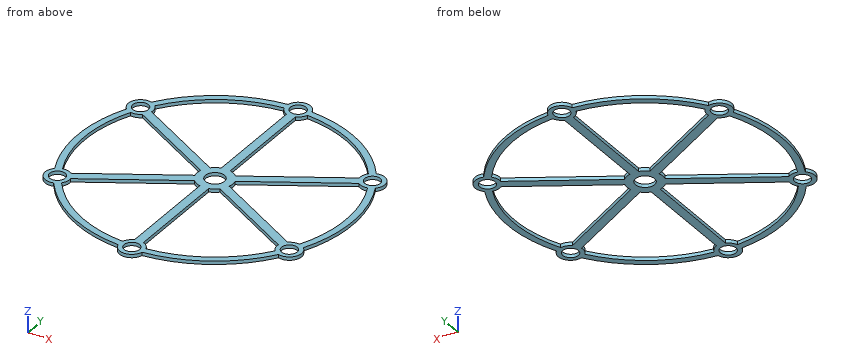
```python
from build123d import *

# Parameters (mm, degrees)
SKETCH_R           = 4.3
SKETCH_R_2         = 3.5
PAD_DEPTH          = 1.5
POLARPATTERN_COUNT = 6


with BuildPart() as part:
    # Sketch → Pad (new body)
    with BuildSketch(Plane.XY):
        with BuildLine():
            ThreePointArc((6.6323005804, 4.4735432278), (4.6158793486, 6.534038402), (2, 7.7459666924))
            Line((2, 7.7459666924), (2, 54.876524617))
            ThreePointArc((2, 54.876524617), (3.9880427931, 56.2124526827), (5.2197393691, 58.2667022995))
            ThreePointArc((48.4987282929, 32.7128052896), (29.7433833833, 50.3744520651), (5.2197393691, 58.2667022995))
            Line((48.4987282929, 32.7128052896), (50.9858410106, 34.390384))
            ThreePointArc((50.9858410106, 34.390384), (31.210195847, 52.9922463235), (5.3521454254, 61.2667041268))
            ThreePointArc((5.3521454254, 61.2667041268), (-3.6080213802, 64.1511663084), (-2, 54.876524617))
            Line((-2, 7.7459666924), (-2, 54.876524617))
            ThreePointArc((-2, 7.7459666924), (-2.8357963608, -7.4805253158), (6.6323005804, 4.4735432278))
        make_face()
        Circle(SKETCH_R, mode=Mode.SUBTRACT)
        with Locations((0, 60)):
            Circle(SKETCH_R_2, mode=Mode.SUBTRACT)
    pad = extrude(amount=PAD_DEPTH)

    # PolarPattern: Pad ×6 about axis
    polarpattern_axis = Axis((0, 0, 0), (0, 0, 1))
    for i in range(1, POLARPATTERN_COUNT):
        add(pad.rotate(polarpattern_axis, i * 360 / POLARPATTERN_COUNT))


solid = part.part
```
Part model, mm, in its own coordinate system. Round coordinates to 2 decimals unless told otherwise and drop trailing zeros. Write each loop counter-clockwise with the first axis right and the second up, starting at its lowest first coordinate (ties: lowest second). Pieces come first, ordered by that corner, then holes. Notation, with made-up numbers: (57.5, 45.5) -> (66.5, 45.5) arc R9 cw to (66.5, 54.5) -> close; hole circle Ø7 at (60.5, -17). An arc over 180 degrees is marked (long way). Return JSON: item names as keys, results as strings. Group by question number.
Q1. Saw through at B-B on x = 32.5. Write the cut outline in (y, z), plus the area to 3 significant figures.
Q2. Pin check, flat tips, straight feed: pin 1 (4 mm diameter, centred on x = -51.96, y = 30, fed in from +Z); pin 2 (0.8 mm diameter, centred on y = 34, z = 1, fed in from -X). Stop position of each tip, or through.
Q3. Saw through at D-D on y = 18.5. Write the cut outline in (x, z).
Q4. Saw through at C-C on y = -46. Write the cut outline in (x, z).
Q5. Probe L1, parallel to Y at x = 51.5, z = 0.7; L2, parallel to Y at x = -36.5, z = 1.35; L3, parallel to X at y = 9.5, z = 0.85. List the from-to ranges inside material, lowest first. Write a range as [from, to].
Q6. Saw through at A-A on y = 0. Write the cut outline in (x, z).
Answer:
{
 "1": {"outline": "(-52.21, 0) -> (-48.64, 0) -> (-48.64, 1.5) -> (-52.21, 1.5) -> close; (-21.07, 0) -> (-16.45, 0) -> (-16.45, 1.5) -> (-21.07, 1.5) -> close; (16.45, 0) -> (21.07, 0) -> (21.07, 1.5) -> (16.45, 1.5) -> close; (48.64, 0) -> (52.21, 0) -> (52.21, 1.5) -> (48.64, 1.5) -> close", "area": "24.6 mm2"},
 "2": {"pin 1": "through", "pin 2": "x = -56.12"},
 "3": {"outline": "(-58.65, 0) -> (-55.5, 0) -> (-55.5, 1.5) -> (-58.65, 1.5) -> close; (-36.04, 0) -> (-28.04, 0) -> (-28.04, 1.5) -> (-36.04, 1.5) -> close; (-2, 0) -> (2, 0) -> (2, 1.5) -> (-2, 1.5) -> close; (28.04, 0) -> (36.04, 0) -> (36.04, 1.5) -> (28.04, 1.5) -> close; (55.5, 0) -> (58.65, 0) -> (58.65, 1.5) -> (55.5, 1.5) -> close"},
 "4": {"outline": "(-40.82, 0) -> (-36.14, 0) -> (-36.14, 1.5) -> (-40.82, 1.5) -> close; (-2, 0) -> (2, 0) -> (2, 1.5) -> (-2, 1.5) -> close; (36.14, 0) -> (40.82, 0) -> (40.82, 1.5) -> (36.14, 1.5) -> close"},
 "5": {"L1": "[-35.48, -33.47], [-26.53, -24.52], [24.52, 26.53], [33.47, 35.48]", "L2": "[-49.5, -45.72], [-23.38, -18.76], [18.76, 23.38], [45.72, 49.5]", "L3": "[-60.76, -57.72], [-20.45, -12.45], [-2, 2], [12.45, 20.45], [57.72, 60.76]"},
 "6": {"outline": "(-61.5, 0) -> (-58.5, 0) -> (-58.5, 1.5) -> (-61.5, 1.5) -> close; (-8, 0) -> (-4.3, 0) -> (-4.3, 1.5) -> (-8, 1.5) -> close; (4.3, 0) -> (8, 0) -> (8, 1.5) -> (4.3, 1.5) -> close; (58.5, 0) -> (61.5, 0) -> (61.5, 1.5) -> (58.5, 1.5) -> close"}
}
